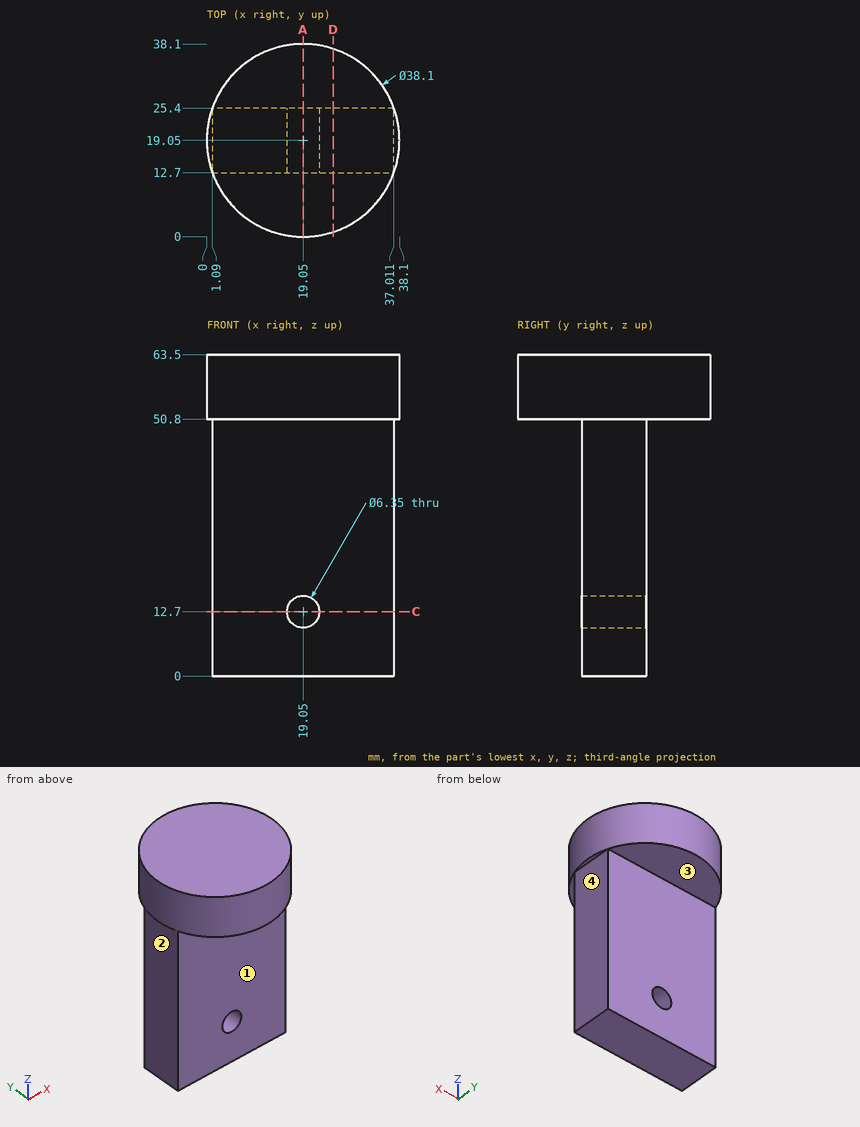
Input: dimensioned drawing with shaded views. Units: mm. Origin: part minimum x, y, z. A direction names the side the tool comes from. Give positions to 0.01 mm unless a question says otherwise; leave off trailing zeros. Write each loop counter-clockwise with the first axis right and the second up, starting at its lowest first coordinate (ties: lowest second). Pieces come first, ordered by that corner, then holes. Notation, with made-up numbers: (-27, 56.5) - (12, 56.5) arc R25 cw to (12, 95.5) - close; hole circle Ø11 at (-20.5, 69.5). An arc over 180 degrees is marked (long way). Write item = value, one per line. Start each with the question number.
1) Cut plane A-A (x = 19.05). Return loops of the section in (y, z) (1 decimal).
2) Cut plane D-D (x = 25). Return loops of the section in (y, z), and give its area (4 significant figures).
3) Pin query (flat end, axial travel): pin 1 (1.2 mm diameter, centred on x = 37.5, y = 16.5, fed in from -Z); pin 2 (4 mm diameter, centred on x = 21, z = 14, fed in from -Y); pin 3 (4 mm diameter, centred on x = 29, z = 19.5, fed in from +Y); pin 4 (10 mm diameter, centred on x = 24, y = 5.5, fed in from -Z). Return the tip coordinate at first contact, or that it passes through.
4) Material intervals for L1, parallel to Z at x = 19, y = 17 (1 decimal); L2, parallel to Z at x = 12, y = 5.5; L3, parallel to X at y = 16.75, z = 12.7 (1 decimal), sorted ascending. Write a range as [from, to].
5) Cut plane C-C (z = 12.7). Return loops of the section in (x, y) (1 decimal).
6) Reachability of the marked faces 1, 2, 3 and 4 from +Z, -Z, +X, -X, +Y, -Y: full face, straight path, thin tool, end or side. Return the list, or none.
Answers follow:
q1.outline = (0, 50.8) - (12.7, 50.8) - (12.7, 15.9) - (25.4, 15.9) - (25.4, 50.8) - (38.1, 50.8) - (38.1, 63.5) - (0, 63.5) - close; (12.7, 0) - (25.4, 0) - (25.4, 9.5) - (12.7, 9.5) - close
q2.outline = (0.95, 50.8) - (12.7, 50.8) - (12.7, 0) - (25.4, 0) - (25.4, 50.8) - (37.15, 50.8) - (37.15, 63.5) - (0.95, 63.5) - close
q2.area = 1,105 mm^2
q3.pin_1 = 0
q3.pin_2 = 12.7
q3.pin_3 = 25.4
q3.pin_4 = 50.8
q4.L1 = [0, 9.5], [15.9, 63.5]
q4.L2 = [50.8, 63.5]
q4.L3 = [1.1, 15.9], [22.2, 37]
q5.outline = (1.1, 12.7) - (15.9, 12.7) - (15.9, 25.4) - (1.1, 25.4) - close; (22.2, 12.7) - (37, 12.7) - (37, 25.4) - (22.2, 25.4) - close
q6.face_1 = -Z, +X, -X, -Y
q6.face_2 = -Z, -X, +Y, -Y
q6.face_3 = -Z, +X, -X, +Y
q6.face_4 = -Z, +X, +Y, -Y
